CAD build for the part. Positions are in the model's coordinates, mm. Face numbers are marked on the shaded views. A direction names the side the tool comes from. Round coordinates to 2 decimals unless told otherwise and drop trailing zeros. Order: outer loops, then holes, each group sorted by start corner. A loop starts at its lowest first (then second) coordinate and runs counter-clockwise, first axis right, second up. Notation, with made-up numbers: M -7.5,57.5 L 20.5,57.5 A11 ccw 20.5,65.5 Z; hole C -8,21 d10. An arc over 180 degrees is marked long. Answer as a JSON object with one key per item and string values. Group by question number.
```python
from build123d import *

# Parameters (mm, degrees)
BOSS_EXTRUDE1_DEPTH      = 75
BOSS_EXTRUDE1_DEPTH_BACK = 75
SKETCH1_W                = 15
SKETCH1_H                = 150
BOSS_EXTRUDE2_DEPTH      = 45
BOSS_EXTRUDE2_DEPTH_BACK = 25
SKETCH2_R                = 13.5
F_20_0MM_DOWEL_HOLE1_D   = 20
FILLET2_R                = 80
FILLET3_R                = 40


with BuildPart() as part:
    # Sketch1 → Boss-Extrude1 (new, two sides: drawn at the far end of the back side and taken through both)
    with BuildSketch(Plane.XY.offset(-BOSS_EXTRUDE1_DEPTH_BACK)):
        Rectangle(SKETCH1_W, SKETCH1_H)
    extrude(amount=BOSS_EXTRUDE1_DEPTH + BOSS_EXTRUDE1_DEPTH_BACK)

    # Sketch2 → Boss-Extrude2 (add, two sides: drawn at the far end of the back side and taken through both)
    with BuildSketch(Plane(origin=(7.5, 0, 0), x_dir=(0, 0, -1), z_dir=(1, 0, 0)).offset(-BOSS_EXTRUDE2_DEPTH_BACK)):
        with Locations((0, -45)):
            Circle(SKETCH2_R)
        with Locations((-45, 45)):
            Circle(SKETCH2_R)
        with Locations((45, 45)):
            Circle(SKETCH2_R)
    extrude(amount=BOSS_EXTRUDE2_DEPTH + BOSS_EXTRUDE2_DEPTH_BACK)

    # Ø20.0mm Dowel Hole1 (through all)
    with Locations(Plane(origin=(52.5, 0, 0), x_dir=(0, 0, -1), z_dir=(1, 0, 0))):
        with Locations((-45, 45), (45, 45), (0, -45)):
            Hole(F_20_0MM_DOWEL_HOLE1_D / 2)

    # Fillet2
    # the kernel refuses this fillet: 80 mm, written as the material it takes off along each edge
    with BuildSketch(Plane(origin=(207.5, -75, -75), x_dir=(0, 0, 1), z_dir=(-1, 0, 0))) as fillet2_piece_1:
        with BuildLine():
            CenterArc((FILLET2_R, FILLET2_R), FILLET2_R, 180, 90)
            Line((0, FILLET2_R), (0, 0))
            Line((0, 0), (FILLET2_R, 0))
        make_face()
    extrude(amount=415, mode=Mode.SUBTRACT)
    with BuildSketch(Plane(origin=(207.5, -75, 75), x_dir=(0, 0, -1), z_dir=(-1, 0, 0))) as fillet2_piece_2:
        with BuildLine():
            CenterArc((FILLET2_R, -FILLET2_R), FILLET2_R, 90, 90)
            Line((0, -FILLET2_R), (0, 0))
            Line((0, 0), (FILLET2_R, 0))
        make_face()
    extrude(amount=415, mode=Mode.SUBTRACT)

    # Fillet3
    fillet3_edges = [part.edges().sort_by_distance(p)[0] for p in [
        (0, 75, 75),
        (0, 75, -75),
    ]]
    fillet(fillet3_edges, radius=FILLET3_R)


solid = part.part
```
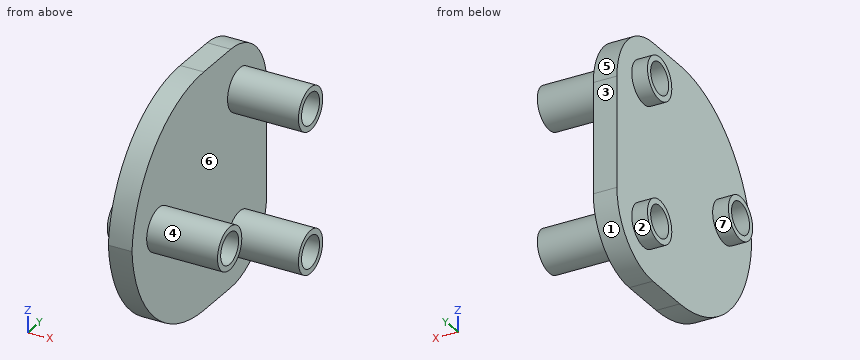
Item 1: Cut at A-A, the plane x = 30. Give the cut face in (y, z), and give its area (3 significant figures).
Item 2: Cut at C-C, the plane z = -45. Give the cut face in (x, y).
Item 3: Drill centre lines: line 1 (Y direction, x = 35, z = 0); line 2 (Z direction, x = 19, y = 50.5); line 3 (X direction, y = 59, z = 1). Where is each one in solid material? Low to high. Write a range as [from, to].
Item 4: Cut at D-D, the plane y = 7.5. Give the cut face in (x, z), and give its area (3 significant figures).
Item 5: Two-plate mould, pull along Z, no slides. Class the marked faces 1, 2, 3 and 4: +Z half, -Z half, draft (parallel to the pull), parting line (faces both ways), or undercut.
Item 6: Flat gauge pins, fed straight in: pin 1 Ø10 at (x, z) = (17, 11.5) entering from +Y; pin 2 Ø2 at (y, z) = (-35, 37.5) entering from -X; pin 3 Ø4 at (x, z) = (17.5, -2) entering from +Y. Where does each tip first touch, or does it go through?
Item 7: Cut at B-B, the plane y = 45. Give the cut face in (x, z), and give its area (3 significant figures).
Item 8: 3-axis set-ups, long thin cutter, end or side, ignore diameter. For the marked faces 5, 6 and 7: which of +Z, -Z, +X, -X, +Y, -Y reach the whole face in a straight line?
Response values:
{
 "1": {"outline": "C -45,0 d27; C 45,-45 d27; C 45,45 d27; hole C -45,0 d20; hole C 45,-45 d20; hole C 45,45 d20", "area": "775 mm^2"},
 "2": {"outline": "M -17.5,31.5 L -7.5,31.5 L -7.5,-57.45 L 7.5,-57.45 L 7.5,31.5 L 52.5,31.5 L 52.5,35 L -17.5,35 Z; M -17.5,55 L 52.5,55 L 52.5,58.5 L 7.5,58.5 L 7.5,73.73 L -7.5,73.73 L -7.5,58.5 L -17.5,58.5 Z"},
 "3": {"line 1": "[-58.5, -55], [-35, -31.5]", "line 2": "[-57.33, -53.35], [-36.65, -32.67], [32.67, 36.65], [53.35, 57.33]", "line 3": "[-7.5, 7.5]"},
 "4": {"outline": "M -7.5,-75 L 7.5,-75 L 7.5,75 L -7.5,75 Z", "area": "2,250 mm^2"},
 "5": {"face 1": "-Z half", "face 2": "undercut", "face 3": "draft", "face 4": "parting line"},
 "6": {"pin 1": "y = -33.17", "pin 2": "x = -7.5", "pin 3": "y = -31.5"},
 "7": {"outline": "M -17.5,-58.5 L -7.5,-58.5 L -7.5,-73.73 L 7.5,-73.73 L 7.5,-58.5 L 52.5,-58.5 L 52.5,-55 L -17.5,-55 Z; M -17.5,-35 L 52.5,-35 L 52.5,-31.5 L 7.5,-31.5 L 7.5,31.5 L 52.5,31.5 L 52.5,35 L -17.5,35 L -17.5,31.5 L -7.5,31.5 L -7.5,-31.5 L -17.5,-31.5 Z; M -17.5,55 L 52.5,55 L 52.5,58.5 L 7.5,58.5 L 7.5,73.73 L -7.5,73.73 L -7.5,58.5 L -17.5,58.5 Z", "area": "2,380 mm^2"},
 "8": {"face 5": "+Z, +X, -X, +Y", "face 6": "+X", "face 7": "-X"}
}
